Autodesk Inventor part; units mm, degrees
ref_plane "YZ Plane" through (0, 0, 0) normal (1, 0, 0) x (0, 1, 0)
ref_plane "XZ Plane" through (0, 0, 0) normal (0, 1, 0) x (-1, 0, 0)
ref_plane "XY Plane" through (0, 0, 0) normal (0, 0, 1) x (1, 0, 0)
sketch "Sketch1" plane through (0, 0, 0) normal (0, 0, 1) x (1, 0, 0)
  line L0 (8.5, -36.236) -> (-8.5, -36.236)
  line L1 (-8.5, -36.236) -> (-8.5, 36.236)
  line L2 (-8.5, 36.236) -> (8.5, 36.236)
  line L3 (8.5, 36.236) -> (8.5, -36.236)
  line L4 (8.5, -36.236) -> (-8.5, 36.236) construction
  line L5 (-8.5, -36.236) -> (8.5, 36.236) construction
  line L6 (8.5, 0) -> (2.5, 0) construction
  line L7 (8.5, 2.75) -> (2.5, 2.75)
  line L8 (2.5, -2.75) -> (8.5, -2.75)
  arc A0 (8.5, -2.75) -> (8.5, 2.75) centre (8.5, 0) ccw
  arc A1 (2.5, 2.75) -> (2.5, -2.75) centre (2.5, 0) ccw
  line L9 (8.5, 36.236) -> (-0.25, 36.236)
  line L10 (-0.25, 36.236) -> (-0.25, 31.236)
  line L11 (2.5, 28.486) -> (8.5, 28.486)
  line L12 (8.5, 28.486) -> (8.5, 36.236)
  line L13 (8.5, -36.236) -> (-0.25, -36.236)
  line L14 (-0.25, -36.236) -> (-0.25, -31.236)
  line L15 (2.5, -28.486) -> (8.5, -28.486)
  line L16 (8.5, -28.486) -> (8.5, -36.236)
  arc A2 (2.5, -28.486) -> (-0.25, -31.236) centre (2.5, -31.236) ccw
  arc A3 (-0.25, 31.236) -> (2.5, 28.486) centre (2.5, 31.236) ccw
  line L17 (0.5, 22.5) -> (0.5, -22.5) construction
  point P0 (0, 0)
  point P1 (5.5, 0)
  point P2 (0.5, 0)
  point P3 (-8.5, 0)
  point P4 (8.5, -28.486)
  point P5 (8.5, 28.486)
  point P6 (-4.5, 0)
  dimension "d0" = 17
  dimension "d1" = 72.472
  dimension "d3" = 5.5
  dimension "d4" = 11
  dimension "d6" = 5
  dimension "d7" = 5
  dimension "d8" = 45
  dimension "d9" = 9
  dimension "d22" = 4
extrude "Extrusion1" add sketch "Sketch1" along normal blind 1.5875 contours L0 L1 L2 L10 A3 L11 L3 L7 A1 L8 L15 A2 L14
fillet "Fillet1" radius 2 2 edges at (-8.5, -36.236, 0.7937) (-8.5, 36.236, 0.7937)
fillet "Fillet2" radius 2 2 edges at (-0.25, -36.236, 0.7937) (-0.25, 36.236, 0.7937)
fillet "Fillet3" radius 1 4 edges at (8.5, -28.486, 0.7937) (8.5, -2.75, 0.7937) (8.5, 2.75, 0.7937) (8.5, 28.486, 0.7937)
hole "Hole1" at (0.5, 22.5, 0) at (0.5, -22.5, 0) direction (0, 0, 1) diameter 3.2 end through all
hole "Hole2" at (-4.5, 0, 0) direction (0, 0, 1) diameter 2.459 end through all
equation "\"d7\" = d6"
properties part number "Gantry Belt Retainer" material "Aluminum 6061"
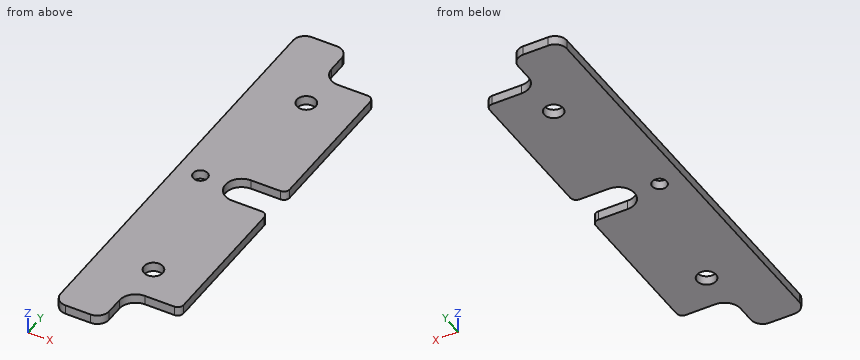
CAD build for the part. Positions are in the model's coordinates, mm. Coordinates: 2 decimals unless noted, no trailing zeros. Order: outer loops, then holes, each group sorted by start corner. A loop starts at its lowest first (then second) coordinate and runs counter-clockwise, first axis right, second up. Notation, with made-up numbers: (-20, 88) -> (-11, 88) arc R18 ccw to (-11, 109) -> close; hole circle Ø5 at (42, -8.75). An arc over 180 degrees is marked (long way). Use one line per item in the form item = value. Start each with the question number.
1) Band-saw the part on A-A on y = 0. Give the cut face in (x, z), then the cut area to 3 significant figures.
2) Drill centre lines: L1, parallel to Y at x = 6, z = 1.4; L2, parallel to Y at x = -4.5, z = 1.1; L3, parallel to X at y = -22.5, z = 0.7. Where is each one in solid material? Low to high. Write a range as [from, to].
3) Band-saw the part on C-C on z = 0.5. Give the cut face in (x, y), then the cut area to 3 significant figures.
4) Band-saw the part on B-B on x = -4.5. Give the cut face in (y, z), then the cut area to 3 significant figures.
5) Drop flat-ended pins along their axis: pin 1 (0.8 mm diameter, centred on x = 4.5, z = 1, fed in from +Y); pin 2 (0.5 mm diameter, centred on x = 6, z = 1, fed in from -Y); pin 3 (0.8 mm diameter, centred on y = 32.5, z = 1, fed in from +X); pin 4 (2 mm diameter, centred on x = -4.5, y = 0, fed in from +Z). Give the stop position or say it passes through.
Entries:
q1.outline = (-8.5, 0) -> (-5.73, 0) -> (-5.73, 1.59) -> (-8.5, 1.59) -> close; (-3.27, 0) -> (-0.25, 0) -> (-0.25, 1.59) -> (-3.27, 1.59) -> close
q1.area = 9.19 mm2
q2.L1 = [-28.49, -2.75], [2.75, 28.49]
q2.L2 = [-36.24, -1.23], [1.23, 36.24]
q2.L3 = [-8.5, -1.1], [2.1, 8.5]
q3.outline = (-8.5, -34.24) arc R2 ccw to (-6.5, -36.24) -> (-2.25, -36.24) arc R2 ccw to (-0.25, -34.24) -> (-0.25, -31.24) arc R2.75 cw to (2.5, -28.49) -> (7.5, -28.49) arc R1 ccw to (8.5, -27.49) -> (8.5, -3.75) arc R1 ccw to (7.5, -2.75) -> (2.5, -2.75) arc R2.75 cw to (2.5, 2.75) -> (7.5, 2.75) arc R1 ccw to (8.5, 3.75) -> (8.5, 27.49) arc R1 ccw to (7.5, 28.49) -> (2.5, 28.49) arc R2.75 cw to (-0.25, 31.24) -> (-0.25, 34.24) arc R2 ccw to (-2.25, 36.24) -> (-6.5, 36.24) arc R2 ccw to (-8.5, 34.24) -> close; hole circle Ø2.46 at (-4.5, 0); hole circle Ø3.2 at (0.5, -22.5); hole circle Ø3.2 at (0.5, 22.5)
q3.area = 1,030 mm2
q4.outline = (-36.24, 0) -> (-1.23, 0) -> (-1.23, 1.59) -> (-36.24, 1.59) -> close; (1.23, 0) -> (36.24, 0) -> (36.24, 1.59) -> (1.23, 1.59) -> close
q4.area = 111 mm2
q5.pin_1 = 28.49
q5.pin_2 = -28.49
q5.pin_3 = -0.25
q5.pin_4 = through
